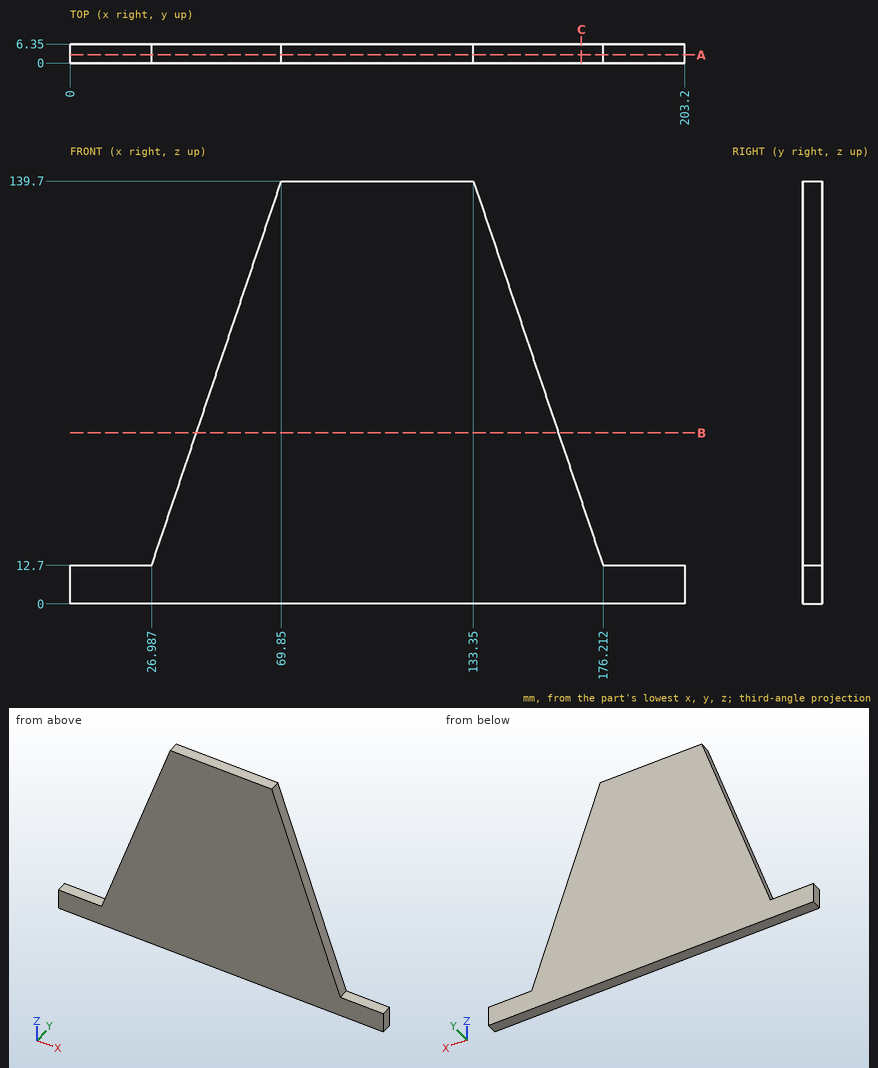
Design review of the part shown in the three views and the two pictorial views. Dimensions are in mm from the part's minimum x, y and z. Give positions to 0.01 mm unless a question says otherwise; leave off trailing zeros. Write each loop counter-clockwise with the first axis right and the second up, starting at its lowest first coordinate (ties: lowest second). Pieces come first, ordered by that corner, then holes. Notation, with made-up numbers: M -10.75,52.25 L 23.25,52.25 A17 ccw 23.25,85.25 Z; hole C -16,-25 d7. An arc over 180 degrees is marked long. One line per question, with ' | ' between items. Start each with the question number.
Item 1: Wall thickness on line 1 (Z direction, x = 25.5, y = 5); line 2 (X direction, y = 2.25, z = 47) (1 decimal); line 3 (X direction, y = 3.5, z = 31.5): over which ranges is each line inside the solid? List them lowest first. Write a range as from..to.
Item 2: For pin 1 (3 mm diameter, centred on x = 196, y = 3.5, fed in from +Z); pin 2 (3 mm diameter, centred on y = 5.5, z = 101, fed in from -X), all flat-tipped, find the tip position at first contact; note any pin that passes through.
Item 3: We need section A-A on y = 2.75. Write out the cut boundary in (x, z), plus the area to 3 significant figures.
Item 4: We need section C-C on x = 169. Write out the cut boundary in (y, z), plus the area to 3 significant figures.
Item 5: We need section B-B on z = 56.5. Write out the cut boundary in (x, y), plus the area to 3 significant figures.
Results found:
1) line 1: z = 0..12.7 | line 2: x = 38.6..164.6 | line 3: x = 33.33..169.87
2) pin 1: stops at z = 12.7 | pin 2: stops at x = 56.28
3) outline: M 0,0 L 203.2,0 L 203.2,12.7 L 176.21,12.7 L 133.35,139.7 L 69.85,139.7 L 26.99,12.7 L 0,12.7 Z | area: 16,100 mm2
4) outline: M 0,0 L 6.35,0 L 6.35,34.07 L 0,34.07 Z | area: 216 mm2
5) outline: M 41.77,0 L 161.43,0 L 161.43,6.35 L 41.77,6.35 Z | area: 760 mm2
